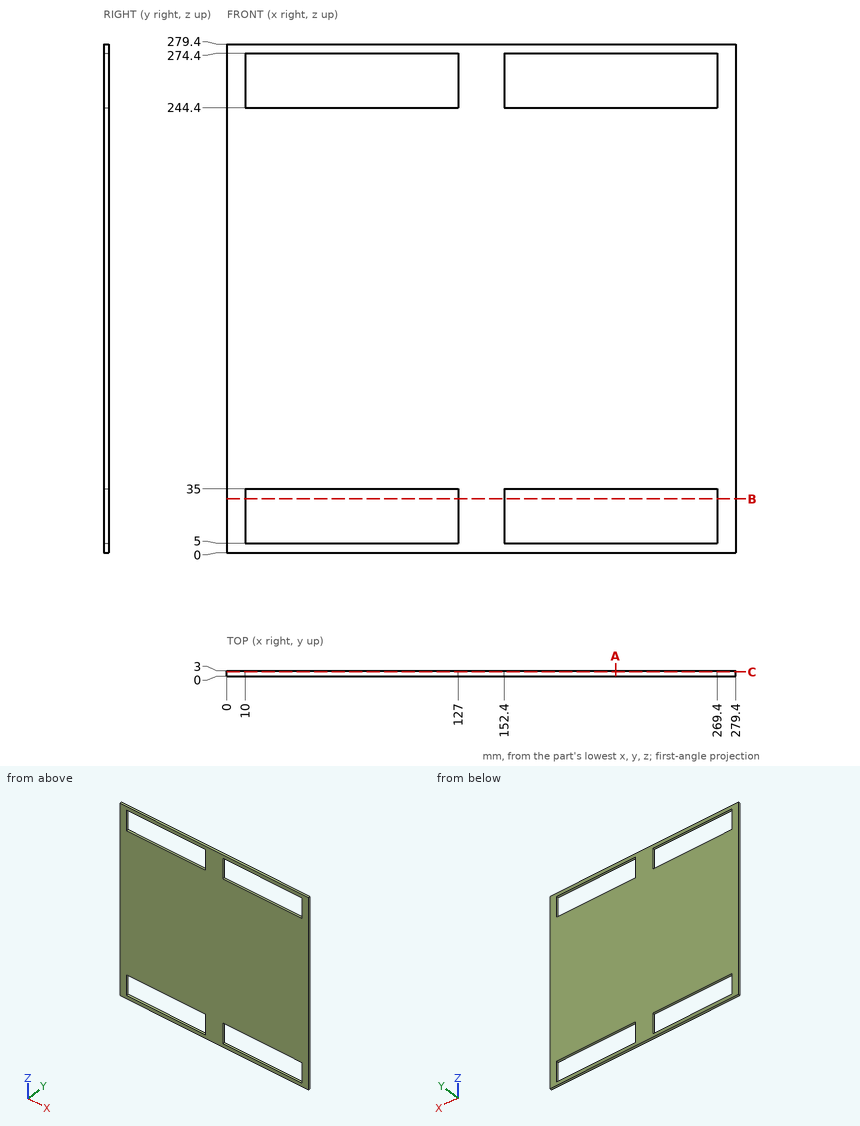
Geometry: see drawing. Coordinates: mm, zero at the bounding-box minimum. Round coordinates to 2 decimals unless told otherwise and drop trailing zeros. Order: outer loops, then holes, each group sorted by start corner. A loop starts at its lowest first (then second) coordinate and runs counter-clockwise, first axis right, second up. Notation, with made-up numbers: (4, 9.25) -> (44, 9.25) arc R18 cw to (44, 39.25) -> close; hole circle Ø9 at (-24.5, -36). An arc over 180 degrees is marked (long way). Answer as CSV lines item,"result".
Item 1: Pin query (flat end, axial travel): pin 1 Ø1.5 at (x, y) = (77.5, 1.5) entering from -Z. Return the tip coordinate at first contact, or that it passes through.
A:
pin 1,"z = 0"
Item 2: Section C-C, the plane y = 2.3. Return loops of the section in (x, z).
A:
outline,"(0, 0) -> (279.4, 0) -> (279.4, 279.4) -> (0, 279.4) -> close; hole (10, 5) -> (127, 5) -> (127, 35) -> (10, 35) -> close; hole (10, 244.4) -> (127, 244.4) -> (127, 274.4) -> (10, 274.4) -> close; hole (152.4, 5) -> (269.4, 5) -> (269.4, 35) -> (152.4, 35) -> close; hole (152.4, 244.4) -> (269.4, 244.4) -> (269.4, 274.4) -> (152.4, 274.4) -> close"
Item 3: Section A-A, the plane x = 213.5. Return loops of the section in (y, z).
A:
outline,"(0, 0) -> (3, 0) -> (3, 5) -> (0, 5) -> close; (0, 35) -> (3, 35) -> (3, 244.4) -> (0, 244.4) -> close; (0, 274.4) -> (3, 274.4) -> (3, 279.4) -> (0, 279.4) -> close"
Item 4: Line query: L1, parallel to Z at x = 63, y = 1.2. Output: solid intervals per line, ascending.
A:
L1,"0 to 5, 35 to 244.4, 274.4 to 279.4"
Item 5: Section B-B, the plane z = 29.5. Return loops of the section in (x, y), plus the area to 3 significant figures.
A:
outline,"(0, 0) -> (10, 0) -> (10, 3) -> (0, 3) -> close; (127, 0) -> (152.4, 0) -> (152.4, 3) -> (127, 3) -> close; (269.4, 0) -> (279.4, 0) -> (279.4, 3) -> (269.4, 3) -> close"
area,"136 mm²"
